```python
from build123d import *

# Parameters (mm, degrees)
SKETCH1_R           = 76.2
BOSS_EXTRUDE1_DEPTH = 38.1
FILLET1_R           = 6.35
CUT_EXTRUDE2_DEPTH  = 39.1
SKETCH3_R           = 57.15
SKETCH3_R_2         = 19.05
CUT_EXTRUDE3_DEPTH  = 6.35


with BuildPart() as part:
    # Sketch1 → Boss-Extrude1 (new body)
    with BuildSketch(Plane.XY):
        Circle(SKETCH1_R)
    extrude(amount=BOSS_EXTRUDE1_DEPTH)

    # Fillet1
    fillet1_edges = [part.edges().sort_by_distance(p)[0] for p in [
        (-76.2, 0, 0),
        (-76.2, 0, 38.1),
    ]]
    fillet(fillet1_edges, radius=FILLET1_R)

    # Sketch2 → Cut-Extrude2 (cut, through all)
    with BuildSketch(Plane.XY.offset(38.1)):
        Polygon((7.332348419, 0), (3.666174209, 6.35), (-3.666174209, 6.35), (-7.332348419, 0), (-3.666174209, -6.35), (3.666174209, -6.35), align=None)
    extrude(amount=-CUT_EXTRUDE2_DEPTH, mode=Mode.SUBTRACT)

    # Sketch3 → Cut-Extrude3 (cut)
    with BuildSketch(Plane.XY.offset(38.1)):
        Circle(SKETCH3_R)
        Circle(SKETCH3_R_2, mode=Mode.SUBTRACT)
    cut_extrude3 = extrude(amount=-CUT_EXTRUDE3_DEPTH, mode=Mode.SUBTRACT)

    # Mirror1: Cut-Extrude3 across plane
    add(cut_extrude3.mirror(Plane.XY.offset(19.05)), mode=Mode.SUBTRACT)


solid = part.part
```
Source: CAD feature listing. Evaluate the final solid. Frame: model axes, mm. A direction names the side the tool comes from. Round coordinates to 2 decimals unless told otherwise and drop trailing zeros. Loops run counter-clockwise (first coordinate to the right, second up) from the corner with the lowest first, then second, coordinate; pieces in that order, holes last. Notation, with made-up numbers: M 27,3.5 L 61,3.5 A21 ccw 61,10.5 Z; hole C 65.25,65.25 d5. An arc over 180 degrees is marked long. Use a Markdown table: item, result. Add a question column.
1. Set-up query: faces 1 (the flat face through (8, 0, 38.1)), 2 (the cylindrical face through (-57.095, 2.513, 34.969)), 3 (the flat face through (-5.525, -3.131, 19.317)), 4 (the cylindrical face through (-57.095, 2.513, 3.131)). Return all of +Z, -Z, +X, -X, +Y, -Y with unobstructed straight access to the full face (end or side cutting, diameter ignored); none if empty.
2. Contact query for flat-ended pins moving along their axis: pin 1 (3 mm diameter, centred on x = -34, z = 22.5, fed in from +Y); pin 2 (10 mm diameter, centred on x = 17.5, z = 14.5, fed in from +Y); pin 3 (1 mm diameter, centred on y = 49, z = 33, fed in from -X). Output: stop coordinate, or through.
3. Cut plane A-A, the plane x = 0. Output: boundary loops of the cut face in (y, z).
4. Pull-direction query (Y, two-part tool) for faces 5 (the cylindrical face through (-60.47, -46.367, 18.872)), 6 (the flat face through (0, 6.35, 19)), 7 (the flat face through (-26.2, -51.4, 0)); classes: +Y half, -Y half, draft (parallel to the pull), parting line (faces both ways), or undercut.
5. Ray query, line 1 along Y through (x, z) = (0, 35.5); line 2 along Z through (x, y) = (0.5, -54.5); line 3 along X through (y, z) = (-6.5, 35.5). Return the intervals inside material, ascending. Write a range as [from, to].
6. Cut plane B-B, the plane z = 27.5. Output: boundary loops of the cut face in (x, y), and give its area (3 significant figures).
Solution:
| question | item | result |
|---|---|---|
| 1 | face 1 | +Z, +X, -X, +Y, -Y |
| 1 | face 2 | +Z |
| 1 | face 3 | +Z, -Z |
| 1 | face 4 | -Z |
| 2 | pin 1 | stops at y = 68.92 |
| 2 | pin 2 | stops at y = 75.17 |
| 2 | pin 3 | stops at x = -58.63 |
| 3 | outline | M -76.2,6.35 A6.35 ccw -69.85,0 L -57.15,0 L -57.15,6.35 L -19.05,6.35 L -19.05,0 L -6.35,0 L -6.35,38.1 L -19.05,38.1 L -19.05,31.75 L -57.15,31.75 L -57.15,38.1 L -69.85,38.1 A6.35 ccw -76.2,31.75 Z; M 6.35,0 L 19.05,0 L 19.05,6.35 L 57.15,6.35 L 57.15,0 L 69.85,0 A6.35 ccw 76.2,6.35 L 76.2,31.75 A6.35 ccw 69.85,38.1 L 57.15,38.1 L 57.15,31.75 L 19.05,31.75 L 19.05,38.1 L 6.35,38.1 Z |
| 4 | face 5 | parting line |
| 4 | face 6 | undercut |
| 4 | face 7 | draft |
| 5 | line 1 | y = [-74.97, -57.15], [-19.05, -6.35], [6.35, 19.05], [57.15, 74.97] |
| 5 | line 2 | z = [6.35, 31.75] |
| 5 | line 3 | x = [-74.69, -56.78], [-17.91, 17.91], [56.78, 74.69] |
| 6 | outline | C 0,0 d152.4; hole M -7.33,0 L -3.67,-6.35 L 3.67,-6.35 L 7.33,0 L 3.67,6.35 L -3.67,6.35 Z |
| 6 | area | 18,100 mm2 |
